Input: part model. Units: mm. Frame: model coordinates. Face numbers are marked on the shaded views. A direction names the side the tool comes from. Round coordinates to 2 decimals unless told otherwise and drop trailing zeros. Loops run counter-clockwise (first coordinate to the right, second up) from the corner with the lowest first, then second, coordinate; pieces in that order, holes last.
(1) Cut plane D-D, the plane z = -15. Output: boundary loops of the cut face in (x, y), and give its area (3 significant figures).
(2) Access query for the marked faces 1 and 2. Directions: +Z, -Z, +X, -X, +Y, -Y. A direction counts if a zero-diameter tool reaches every point of the face in a straight line with its end or side. Return the directions, or none.
(3) Cut plane C-C, the plane x = 9. Output: boundary loops of the cut face in (y, z) (3 decimals).
(4) First-contact query: pin 1 Ø10 at (x, z) = (4, -11.5) entering from +Y. Flat tip, straight axial feed; report the tip coordinate or a pass-through.
(5) Line query: line 1 (X direction, y = 0.3, z = 0.5); line 2 (Z direction, x = 29.5, y = 0.65); line 3 (X direction, y = 0.65, z = 7.5). Output: solid intervals per line, ascending.
(6) Cut plane B-B, the plane z = 5. Output: boundary loops of the cut face in (x, y), and give its area (3 significant figures).
(7) Cut plane A-A, the plane y = -0.3. Output: boundary loops of the cut face in (x, z) (3 decimals), and give its area (3 significant figures).
from build123d import *

# Parameters (mm, degrees)
EXTRUDE_1_DEPTH     = 0.75
SKETCH_2_R          = 2
EXTRUDE_2_DEPTH     = 1.25
SKETCH_3_R          = 1.25
CUT_EXTRUDE_1_DEPTH = 3
SKETCH_4_W          = 42.3
SKETCH_4_H          = 30
CUT_EXTRUDE_2_DEPTH = 3
FILLET_1_R          = 2
CUT_EXTRUDE_3_DEPTH = 1.75


with BuildPart() as part:
    # 草图1 → 凸台-拉伸1 (new body)
    with BuildSketch(Plane(origin=(0, 0, 0), x_dir=(1, 0, 0), z_dir=(0, 1, 0))):
        with BuildLine():
            Line((-28.283443195, 18.335), (28.716556805, 18.335))
            ThreePointArc((28.716556805, 18.335), (32.181380033, 16.899823228), (33.616556805, 13.435))
            Line((33.616556805, 13.435), (33.616556805, -10.765))
            ThreePointArc((33.616556805, -10.765), (32.181380033, -14.229823228), (28.716556805, -15.665))
            Line((28.716556805, -15.665), (20.216556805, -15.665))
            Line((20.216556805, -15.665), (-19.783443195, -15.665))
            Line((-19.783443195, -15.665), (-28.283443195, -15.665))
            ThreePointArc((-28.283443195, -15.665), (-31.748266423, -14.229823228), (-33.183443195, -10.765))
            Line((-33.183443195, -10.765), (-33.183443195, 13.435))
            ThreePointArc((-33.183443195, 13.435), (-31.748266423, 16.899823228), (-28.283443195, 18.335))
        make_face()
    extrude(amount=EXTRUDE_1_DEPTH)

    # 草图2 → 凸台-拉伸2 (add)
    with BuildSketch(Plane.XZ):
        with Locations((-28.783443195, 12.065)):
            Circle(SKETCH_2_R)
        with Locations((-28.783443195, -10.935)):
            Circle(SKETCH_2_R)
        with Locations((29.216556805, 12.065)):
            Circle(SKETCH_2_R)
        with Locations((29.216556805, -10.935)):
            Circle(SKETCH_2_R)
    extrude(amount=EXTRUDE_2_DEPTH)

    # 草图3 → 切除-拉伸1 (cut, through all)
    with BuildSketch(Plane.XZ.offset(1.25)):
        with Locations((-28.783443195, 12.065)):
            Circle(SKETCH_3_R)
        with Locations((-28.783443195, -10.935)):
            Circle(SKETCH_3_R)
        with Locations((29.216556805, -10.935)):
            Circle(SKETCH_3_R)
        with Locations((29.216556805, 12.065)):
            Circle(SKETCH_3_R)
    extrude(amount=-CUT_EXTRUDE_1_DEPTH, mode=Mode.SUBTRACT)

    # 草图4 → 切除-拉伸2 (cut, through all)
    with BuildSketch(Plane(origin=(0, 0.75, 0), x_dir=(1, 0, 0), z_dir=(0, 1, 0))):
        with Locations((1.966556805, -0.665)):
            Rectangle(SKETCH_4_W, SKETCH_4_H)
    extrude(amount=-CUT_EXTRUDE_2_DEPTH, mode=Mode.SUBTRACT)

    # 圆角1
    fillet_1_edges = [part.edges().sort_by_distance(p)[0] for p in [
        (-19.183443195, 0.375, 15.665),
        (-19.183443195, 0.375, -14.335),
        (23.116556805, 0.375, -14.335),
        (23.116556805, 0.375, 15.665),
    ]]
    fillet(fillet_1_edges, radius=FILLET_1_R)

    # 草图6 → 切除-拉伸3 (cut, through all)
    with BuildSketch(Plane.XZ):
        with BuildLine():
            Line((-27.783443195, 2.765), (-24.783443195, 2.765))
            ThreePointArc((-24.783443195, 2.765), (-24.076336414, 2.472106781), (-23.783443195, 1.765))
            Line((-23.783443195, 1.765), (-23.783443195, -0.235))
            ThreePointArc((-23.783443195, -0.235), (-24.076336414, -0.942106781), (-24.783443195, -1.235))
            Line((-24.783443195, -1.235), (-27.783443195, -1.235))
            ThreePointArc((-27.783443195, -1.235), (-28.490549976, -0.942106781), (-28.783443195, -0.235))
            Line((-28.783443195, -0.235), (-28.783443195, 1.765))
            ThreePointArc((-28.783443195, 1.765), (-28.490549976, 2.472106781), (-27.783443195, 2.765))
        make_face()
    extrude(amount=-CUT_EXTRUDE_3_DEPTH, mode=Mode.SUBTRACT)


solid = part.part
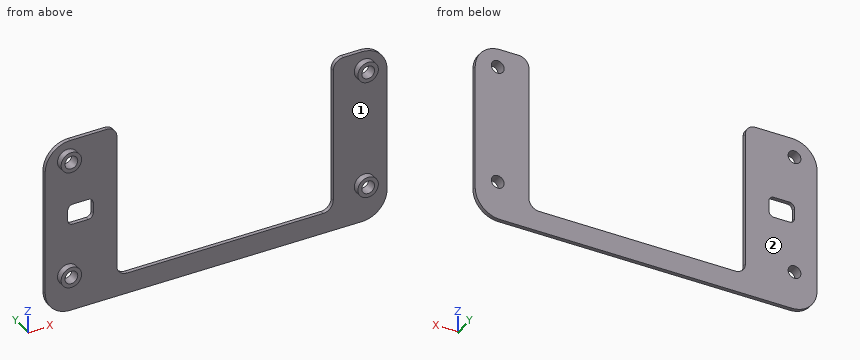
Reported:
1. outline: (-32.93, 0) - (33.36, 0) - (33.36, 0.75) - (-32.93, 0.75) - close
1. area: 49.7 mm2
2. face 1: -Y
2. face 2: +Z, -Z, +X, -X, +Y
3. outline: (0, -18.335) - (0.75, -18.335) - (0.75, -14.335) - (0, -14.335) - close
4. pin 1: stops at y = 0.75
5. line 1: x = -33.18 to -28.78, -23.78 to -19.18, 23.12 to 33.62
5. line 2: z = -18.27 to -12.15, -9.72 to 10.85, 13.28 to 15.6
5. line 3: x = -33.18 to -19.18, 23.12 to 33.62
6. outline: (-33.18, 0) - (-19.18, 0) - (-19.18, 0.75) - (-33.18, 0.75) - close; (23.12, 0) - (33.62, 0) - (33.62, 0.75) - (23.12, 0.75) - close
6. area: 18.4 mm2
7. outline: circle Ø4 at (-28.783, -10.935); circle Ø4 at (-28.783, 12.065); circle Ø4 at (29.217, -10.935); circle Ø4 at (29.217, 12.065); hole circle Ø2.5 at (-28.783, -10.935); hole circle Ø2.5 at (-28.783, 12.065); hole circle Ø2.5 at (29.217, -10.935); hole circle Ø2.5 at (29.217, 12.065)
7. area: 30.6 mm2
